```python
from build123d import *

# Parameters (mm, degrees)
SKETCH001_R       = 43
PAD_DEPTH         = 8
SKETCH002_W       = 5
SKETCH002_H       = 50
SKETCH003_R       = 33
POCKET_DEPTH      = 8.001
POCKET_DEPTH_BACK = 8.001
SKETCH004_W       = 3
SKETCH004_H       = 50


with BuildPart() as part:
    # Sketch001 → Pad (new body, symmetric)
    with BuildSketch(Plane.XZ):
        Circle(SKETCH001_R)
    extrude(amount=PAD_DEPTH, both=True)

    # Sketch002 → Revolution (revolve)
    with BuildSketch(Plane.XZ):
        with Locations((-30.5, 25)):
            Rectangle(SKETCH002_W, SKETCH002_H)
    revolve(axis=Axis((-28, 0, 41.317169), (0, 0, -1)))

    # Sketch003 → Pocket (cut, two sides)
    with BuildSketch(Plane.XZ) as pocket_sk:
        Circle(SKETCH003_R)
    extrude(amount=-POCKET_DEPTH, mode=Mode.SUBTRACT)
    extrude(pocket_sk.sketch, amount=POCKET_DEPTH_BACK, mode=Mode.SUBTRACT)

    # Sketch004 → Groove (revolve, cut)
    with BuildSketch(Plane.XZ):
        with Locations((-26.5, 25)):
            Rectangle(SKETCH004_W, SKETCH004_H)
    revolve(axis=Axis((-28, 0, 41.317169), (0, 0, -1)), mode=Mode.SUBTRACT)


solid = part.part
```
Design review of the part built by this model. Coordinates are the model's own, in mm. A direction names the side the tool comes from. Round coordinates to 2 decimals unless told otherwise and drop trailing zeros. Order: outer loops, then holes, each group sorted by start corner. A loop starts at its lowest first (then second) coordinate and runs counter-clockwise, first axis right, second up. Notation, with made-up numbers: M 88,68 L 136,68 A31 cw 136,106 Z; hole C 38,62.25 d7. An arc over 180 degrees is marked long. Put each result on its own line as item: value.
Q1. Draft analysis for pull direction Y (two halves, no side actions). For faces 3 (the face through (-10, 8, -32)), 4 (the face through (-31, 0, 35)), 5 (the face through (-27.9, -3.3, 50)), state which applies: released by +Y, released by -Y, zero draft, split by the parting line, or undercut.
Reported:
face 3: released by +Y
face 4: undercut
face 5: zero draft
Q2. Consider section D-D (x = -26.5). State the section outline as (y, z) points, and give its area (3 significant figures).
Reported:
outline: M -8,-33.86 L 8,-33.86 L 8,-19.67 L -8,-19.67 Z; M -8,19.67 L -2.6,19.67 L -2.6,50 L -4.77,50 L -4.77,33.86 L -8,33.86 Z; M 2.6,19.67 L 8,19.67 L 8,33.86 L 4.77,33.86 L 4.77,50 L 2.6,50 Z
area: 451 mm²
Q3. To check wall thickness, follow line 1 (Y direction, x = -28, z = 40.5); line 2 (Z direction, x = 0, y = 6.5); line 3 (X direction, y = 0, z = 27.5). State the ranges of each line that lie inside material, in increasing order.
Reported:
line 1: -5 to -3, 3 to 5
line 2: -43 to -33, 33 to 43
line 3: -33.06 to -31, -25 to -18.24, 18.24 to 33.06
Q4. Consider section A-A (z = 0). State the section outline as (x, y) points, and give its area (3 significant figures).
Reported:
outline: M -43,-8 L -33,-8 L -33,8 L -43,8 Z; M 33,-8 L 43,-8 L 43,8 L 33,8 Z
area: 320 mm²
Q5. Consider section B-B (x = 0). State the section outline as (y, z) points, and give its area (3 significant figures).
Reported:
outline: M -8,-43 L 8,-43 L 8,-33 L -8,-33 Z; M -8,33 L 8,33 L 8,43 L -8,43 Z
area: 320 mm²
Q6. Insertion check: pin 1 Ø6 at (x, y) = (-3.5, -4) entering from +Z; pin 2 Ø5 at (x, y) = (-28, 0) entering from +Z; pin 3 Ø1 at (x, y) = (5.5, -4.5) entering from +Z. Each pin has a flat end and moves straight along its axis. Give the tip position at first contact, or say it passes through.
Reported:
pin 1: z = 43
pin 2: z = -12.6
pin 3: z = 42.71
Q7. Consider section C-C (z = 29). State the section outline as (x, y) points.
Reported:
outline: M -31.75,-8 L -15.75,-8 L -15.75,8 L -31.75,8 L -31.75,3.31 A5 ccw -31.75,-3.31 Z; M 15.75,-8 L 31.75,-8 L 31.75,8 L 15.75,8 Z; hole C -28,0 d6
Q8. Machinability: for faces 1 (the face through (-10, -8, -32)), 2 (the face through (-32.619, -1.915, 41.434)), which of the approach directions +Z, -Z, +X, -X, +Y, -Y give a long, thin tool a straight path to every point of the face, cutting with its end or side? Answer none if there is none.
Reported:
face 1: +Z, -Z, +X, -X, -Y
face 2: +Z
